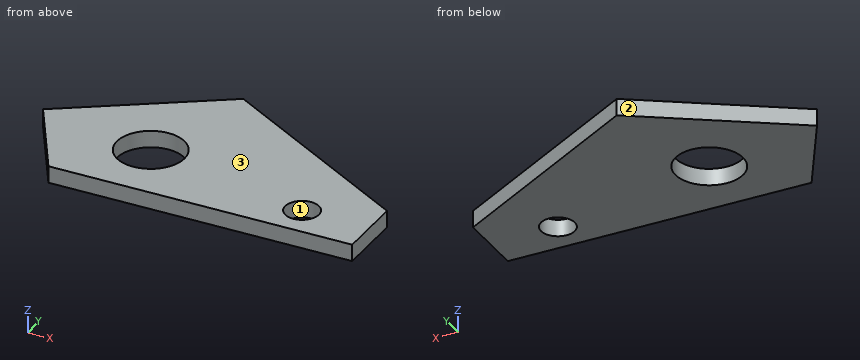
Autodesk Inventor part; units mm, degrees
ref_plane "YZ Plane" through (0, 0, 0) normal (1, 0, 0) x (0, 1, 0)
ref_plane "XZ Plane" through (0, 0, 0) normal (0, 1, 0) x (-1, 0, 0)
ref_plane "XY Plane" through (0, 0, 0) normal (0, 0, 1) x (1, 0, 0)
sketch "Sketch1" plane through (0, 0, 0) normal (0, 0, 1) x (1, 0, 0)
  line L0 (114.3, 0) -> (114.3, 25.4)
  line L1 (114.3, 25.4) -> (37.3103, 69.85)
  line L2 (0, 0) -> (-19.05, 32.9956)
  line L3 (-19.05, 32.9956) -> (37.3103, 69.85)
  circle A0 centre (25.4, 25.4) radius 12.7
  circle A1 centre (88.9, 12.7) radius 6.35
  line L4 (0, 0) -> (114.3, 0)
  dimension "d1" = 25.4
  dimension "d2" = 88.9
  dimension "d4" = 38.1
  dimension "d8" = 25.4
  dimension "d11" = 12.7
extrude "Extrusion1" add sketch "Sketch1" along normal blind 6.35
properties part number "Assignment 1.5 - Slider Block"
Here's how the part is built. I have some questions about the finished solid (model axes, mm). Face numbers are marked on the shaded views. Round coordinates to 2 decimals unless told otherwise and drop trailing zeros. Loops run counter-clockwise (first coordinate to the right, second up) from the corner with the lowest first, then second, coordinate; pieces in that order, holes last.
1. For P1, Ø1, axis at y = 26, z = 3, coming from the -X side, with a flat end and sliding along its axis, tell me the tip position at first contact or that it passes through.
Answer list:
P1: stops at x = -15.3
2. If I drill on line 1 along X through (y, z) = (15.5, 6); line 2 along Y through (x, z) = (88.9, 1.5); line 3 along Y through (x, z) = (31.5, 4.75), over which ranges is the centre line in solid material (lowest first)?
Answer list:
line 1: x = -8.95 to 17.45, 33.35 to 83.2, 94.6 to 114.3
line 2: y = 0 to 6.35, 19.05 to 40.06
line 3: y = 0 to 14.26, 36.54 to 66.05
3. If we section it at A-A on z = 2.25: Write out the boundary of the cut face in (x, y), plus the area to 3 significant figures.
Answer list:
outline: (-19.05, 33) - (0, 0) - (114.3, 0) - (114.3, 25.4) - (37.31, 69.85) - close; hole circle Ø25.4 at (25.4, 25.4); hole circle Ø12.7 at (88.9, 12.7)
area: 5,620 mm2
4. If we section it at C-C on x = 25.4: Write out the boundary of the cut face in (y, z).
Answer list:
outline: (0, 0) - (12.7, 0) - (12.7, 6.35) - (0, 6.35) - close; (38.1, 0) - (62.06, 0) - (62.06, 6.35) - (38.1, 6.35) - close
5. We'd pull the mould along X, two halves only. Please class the marked faces 1, 2 and 3: +X half, -X half, draft (parallel to the pull), parting line (faces both ways), or undercut.
Answer list:
face 1: undercut
face 2: -X half
face 3: draft
6. If we section it at D-D on x = 56.5: Write out the boundary of the cut face in (y, z), plus the area to 3 significant figures.
Answer list:
outline: (0, 0) - (58.77, 0) - (58.77, 6.35) - (0, 6.35) - close
area: 373 mm2
7. If we section it at B-B on y = 23: Write out the boundary of the cut face in (x, z), plus the area to 3 significant figures.
Answer list:
outline: (-13.28, 0) - (12.93, 0) - (12.93, 6.35) - (-13.28, 6.35) - close; (37.87, 0) - (114.3, 0) - (114.3, 6.35) - (37.87, 6.35) - close
area: 652 mm2
